Can you work these out from the model? Positions are in its coordinate system, mm. Round coordinates to 2 decimals unless told otherwise and drop trailing zeros. Loops run counter-clockwise (first coordinate to the right, second up) from the corner with the lowest first, then second, coordinate; pieces in that order, holes last. Notation, with made-up numbers: (89, 37) -> (134, 37) arc R21 ccw to (134, 59) -> close; hole circle Ø7 at (39.5, 48). An arc over 180 degrees is marked (long way). Answer as a JSON object with one key per item and string values.
```python
from build123d import *

# Parameters (mm, degrees)
SKETCH_1_R      = 1.44
SKETCH_1_R_2    = 3.6
EXTRUDE_2_DEPTH = 2
SKETCH_1_2_R    = 1.44
SKETCH_1_2_R_2  = 3.6
EXTRUDE_3_DEPTH = 3.5


with BuildPart() as part:
    # 草图1 → 凸台-拉伸2 (new body)
    with BuildSketch(Plane.XY):
        with BuildLine():
            Line((-15, 6.5), (15, 6.5))
            ThreePointArc((15, 6.5), (21.5, 0), (15, -6.5))
            Line((15, -6.5), (-15, -6.5))
            ThreePointArc((-15, -6.5), (-21.5, 0), (-15, 6.5))
        make_face()
        with Locations((-15, 0)):
            Circle(SKETCH_1_R, mode=Mode.SUBTRACT)
        with Locations((15, 0)):
            Circle(SKETCH_1_R, mode=Mode.SUBTRACT)
        Circle(SKETCH_1_R_2, mode=Mode.SUBTRACT)
    extrude(amount=EXTRUDE_2_DEPTH)

    # 草图1<2> → 凸台-拉伸3 (add)
    with BuildSketch(Plane.XY):
        with BuildLine():
            Line((-15, 6.5), (15, 6.5))
            ThreePointArc((15, 6.5), (21.5, 0), (15, -6.5))
            Line((15, -6.5), (-15, -6.5))
            ThreePointArc((-15, -6.5), (-21.5, 0), (-15, 6.5))
        make_face()
        with Locations((-15, 0)):
            Circle(SKETCH_1_2_R, mode=Mode.SUBTRACT)
        with Locations((15, 0)):
            Circle(SKETCH_1_2_R, mode=Mode.SUBTRACT)
        Circle(SKETCH_1_2_R_2, mode=Mode.SUBTRACT)
    extrude(amount=EXTRUDE_3_DEPTH)


solid = part.part
```
Q1. I'm going to push a flat-ended pin straight in: pin 1 (4.5 mm diameter, centred on x = 0, y = 0, fed in from +Z). Where does the tip first touch, or does it pass through?
Determined:
{"pin 1": "through"}
Q2. If I drill on L1, parallel to Y at x = 15, z = 1.25; L2, parallel to X at y = -1, z = 3.1; L3, parallel to Y at x = 2, z = 1.2, over which ranges is the centre line in solid material (lowest first)? Write a range as [from, to].
Determined:
{"L1": "[-6.5, -1.44], [1.44, 6.5]", "L2": "[-21.42, -16.04], [-13.96, -3.46], [3.46, 13.96], [16.04, 21.42]", "L3": "[-6.5, -2.99], [2.99, 6.5]"}
Q3. I want a section at D-D, the plane x = -17.5. Write out the boundary of the cut face in (y, z), then the cut area to 3 significant figures.
Determined:
{"outline": "(-6, 0) -> (6, 0) -> (6, 3.5) -> (-6, 3.5) -> close", "area": "42.0 mm²"}
Q4. We'd pull the mould along Y, two halves only. Please class faces 1 (the cylindrical face through (-13.67, -0.55, 1.73)), 2 (the flat face through (0, -6.5, 2)), 3 (the cylindrical face through (-21.5, -0.1, 1.7)): pulls with the +Y half, pulls with the -Y half, needs draft (parallel to the pull), parting line crosses it, or undercut.
Determined:
{"face 1": "undercut", "face 2": "pulls with the -Y half", "face 3": "parting line crosses it"}
Q5. I want a section at C-C, the plane z = 1.45. Write out the boundary of the cut face in (x, y).
Determined:
{"outline": "(-15, -6.5) -> (15, -6.5) arc R6.5 ccw to (15, 6.5) -> (-15, 6.5) arc R6.5 ccw to start; hole circle Ø2.88 at (-15, 0); hole circle Ø7.2 at (0, 0); hole circle Ø2.88 at (15, 0)"}
Q6. I want a section at B-B, the plane x = 0. Write out the boundary of the cut face in (y, z).
Determined:
{"outline": "(-6.5, 0) -> (-3.6, 0) -> (-3.6, 3.5) -> (-6.5, 3.5) -> close; (3.6, 0) -> (6.5, 0) -> (6.5, 3.5) -> (3.6, 3.5) -> close"}
Q7. I want a section at A-A, the plane y = 0. Write out the boundary of the cut face in (x, z), then the cut area to 3 significant figures.
Determined:
{"outline": "(-21.5, 0) -> (-16.44, 0) -> (-16.44, 3.5) -> (-21.5, 3.5) -> close; (-13.56, 0) -> (-3.6, 0) -> (-3.6, 3.5) -> (-13.56, 3.5) -> close; (3.6, 0) -> (13.56, 0) -> (13.56, 3.5) -> (3.6, 3.5) -> close; (16.44, 0) -> (21.5, 0) -> (21.5, 3.5) -> (16.44, 3.5) -> close", "area": "105 mm²"}
